```python
from build123d import *

# Parameters (mm, degrees)
BOX001_W                   = 10
BOX001_H                   = 20
BOX001_DEPTH               = 1
BOX004_W                   = 11
BOX004_H                   = 2.6
BOX004_DEPTH               = 8
EXTRUDE003_DEPTH           = 10
EXTRUDE003_PLACEMENT_ANGLE = 90
FUSION003_PLACEMENT_ANGLE  = 270
BOX003_W                   = 10
BOX003_H                   = 1
BOX003_DEPTH               = 4
BOX_W                      = 10
BOX_H                      = 18
BOX_DEPTH                  = 1
BOX002_W                   = 10
BOX002_H                   = 1
BOX002_DEPTH               = 2


with BuildPart() as cube001:
    # Box001 → Box001 (new body)
    with BuildSketch(Plane.XY.offset(3)):
        with Locations((5, 10)):
            Rectangle(BOX001_W, BOX001_H)
    extrude(amount=BOX001_DEPTH)


with BuildPart() as cube004:
    # Box004 → Box004 (new body)
    with BuildSketch(Plane(origin=(0, 5.7, -4), x_dir=(1, 0, 0), z_dir=(0, 0, 1))):
        with Locations((5.5, 1.3)):
            Rectangle(BOX004_W, BOX004_H)
    extrude(amount=BOX004_DEPTH)


with BuildPart() as keymaster:
    # RegularPolygon003 → Extrude003 (new body)
    with BuildSketch(Plane(origin=(-2.737398, 7, 0), x_dir=(0, 1, 0), z_dir=(0, 0, 1))):
        Polygon((0, -2.487398), (2.615405, -0.587195), (1.616409, 2.487398), (-1.616409, 2.487398), (-2.615405, -0.587195), align=None)
    extrude(amount=EXTRUDE003_DEPTH)


with BuildPart() as keymaster_1:
    # Extrude003 placement: moved
    add(keymaster.part.rotate(Axis((0, 0, 0), (0, 1, 0)), EXTRUDE003_PLACEMENT_ANGLE))

    # Fusion003: union Cube004
    add(cube004.part)


with BuildPart() as keymaster_2:
    # Fusion003 placement: moved
    add(keymaster_1.part.moved(Location((-2, 10, 7))).rotate(Axis((-2, 10, 7), (0, 0, 1)), FUSION003_PLACEMENT_ANGLE))


with BuildPart() as cube003:
    # Box003 → Box003 (new body)
    with BuildSketch(Plane.XY):
        with Locations((5, 0.5)):
            Rectangle(BOX003_W, BOX003_H)
    extrude(amount=BOX003_DEPTH)


with BuildPart() as cube:
    # Box → Box (new body)
    with BuildSketch(Plane.XY):
        with Locations((5, 9)):
            Rectangle(BOX_W, BOX_H)
    extrude(amount=BOX_DEPTH)


with BuildPart() as fusion:
    # Box002 → Box002 (new body)
    with BuildSketch(Plane(origin=(0, 19, 1), x_dir=(1, 0, 0), z_dir=(0, 0, 1))):
        with Locations((5, 0.5)):
            Rectangle(BOX002_W, BOX002_H)
    extrude(amount=BOX002_DEPTH)

    # Fusion: union Cube001, keymaster, Cube003, Cube
    add(cube001.part)
    add(keymaster_2.part)
    add(cube003.part)
    add(cube.part)


solid = fusion.part
```
Model file for the job. Use its own axes, mm. A direction names the side the tool comes from. Coordinates: 2 decimals unless noted, no trailing zeros. Loops run counter-clockwise (first coordinate to the right, second up) from the corner with the lowest first, then second, coordinate; pieces in that order, holes last. Notation, with made-up numbers: (72, -25.75) -> (101, -25.75) arc R25 cw to (101, -13.75) -> close; hole circle Ø2 at (84, -19.75). An arc over 180 degrees is marked (long way). Answer as a JSON object with one key per item and string values.
Q1. Cut at C-C (x = 2). List the corners of the cut face in (y, z), and give its area (3 significant figures).
Report:
{"outline": "(0, 0) -> (18, 0) -> (18, 1) -> (1, 1) -> (1, 3) -> (19, 3) -> (19, 1) -> (20, 1) -> (20, 4) -> (0, 4) -> close", "area": "42.0 mm2"}
Q2. 3-axis set-ups, long thin cutter, end or side, ignore diameter. For faces 1 (the flat face through (5, 19, 2)), 2 (the flat face through (3.03, 5.07, 8.68)), 3 (the flat face through (6.948, 5.07, 8.666)), 4 (the flat face through (5, 1, 2)): which of +Z, -Z, +X, -X, +Y, -Y reach the whole face in a straight line?
Report:
{"face 1": "-Z, +X, -X", "face 2": "-X, +Y, -Y", "face 3": "+X, +Y, -Y", "face 4": "+X, -X"}
Q3. Cut at A-A (y = 13). List the corners of the cut face in (x, z), and give its area (3 significant figures).
Report:
{"outline": "(0, 0) -> (10, 0) -> (10, 1) -> (0, 1) -> close; (0, 3) -> (10, 3) -> (10, 4) -> (0, 4) -> close", "area": "20.0 mm2"}
Q4. Pull direction Y, two halves, no side cores. Call faces 5 (the flat face through (5, 20, 2)), 6 (the flat face through (3.7, 5, 6)), 7 (the flat face through (5, 10, 1)): released by +Y, released by -Y, zero draft, split by the parting line, or undercut.
Report:
{"face 5": "released by +Y", "face 6": "zero draft", "face 7": "undercut"}
Q5. Flat gauge pins, fed straight in: P1, Ø2.5, axis at y = 3.5, z = 6.5, coming from the +X side; P2, Ø0.6, axis at x = 4, z = 2.5, coming from the -Y side; P3, Ø2.5, axis at y = 6, z = 6, coming from the -X side. Where does each tip first touch, or does it go through?
Report:
{"P1": "stops at x = 6.3", "P2": "stops at y = 0", "P3": "stops at x = 3.7"}
Q6. Probe probe 1 along Z at (x, y) = (4.5, 7.75); probe 2 along Z at (x, y) = (6.75, 11.5); probe 3 along Y at (x, z) = (8, 1.5). List the from-to ranges inside material, lowest first.
Report:
{"probe 1": "z = 0 to 1, 3 to 12.22", "probe 2": "z = 0 to 1, 3 to 4", "probe 3": "y = 0 to 1, 19 to 20"}
Q7. Cut at D-D (z = 3.25). List the corners of the cut face in (x, y).
Report:
{"outline": "(0, 0) -> (3.7, 0) -> (3.7, -1) -> (6.3, -1) -> (6.3, 0) -> (10, 0) -> (10, 20) -> (0, 20) -> close"}
Q8. Cut at B-B (z = 1.5). List the corners of the cut face in (x, y).
Report:
{"outline": "(0, 0) -> (10, 0) -> (10, 1) -> (0, 1) -> close; (0, 19) -> (10, 19) -> (10, 20) -> (0, 20) -> close"}
